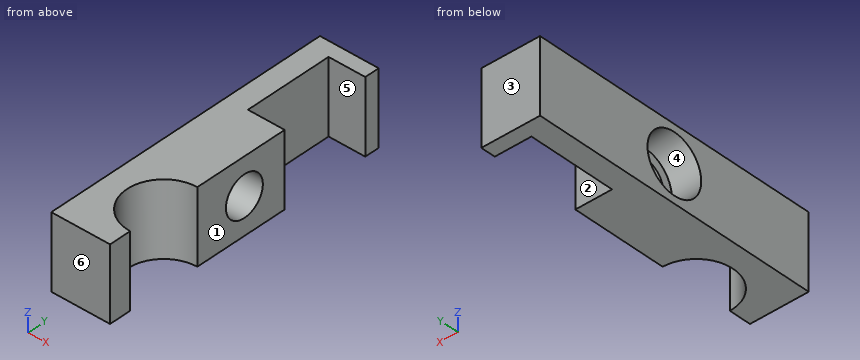
Autodesk Inventor part; units mm, degrees
ref_plane "YZ Plane" through (0, 0, 0) normal (1, 0, 0) x (0, 1, 0)
ref_plane "XZ Plane" through (0, 0, 0) normal (0, 1, 0) x (-1, 0, 0)
ref_plane "XY Plane" through (0, 0, 0) normal (0, 0, 1) x (1, 0, 0)
sketch "Sketch1" plane through (0, 0, 0) normal (0, 0, 1) x (1, 0, 0)
  line L0 (0, 0) -> (4, 0)
  line L1 (4, 0) -> (4, -20)
  line L2 (4, -20) -> (0, -20)
  line L3 (0, -20) -> (0, 0)
  circle A0 centre (4, -4) radius 2.5
  circle A1 centre (4, -16) radius 2.5
  line L4 (1.5, -4) -> (1.5, -7)
  line L5 (1.5, -7) -> (1.5, -1)
  line L6 (4, -7) -> (1.5, -7)
  line L7 (1.5, -1) -> (4, -1)
  point P0 (4, -18.5)
  point P1 (4, -13.5)
  dimension "d2" = 5
  dimension "d0" = 20
  dimension "d1" = 4
  dimension "d3" = 5
  dimension "d4" = 4
  dimension "d5" = 4
  dimension "d6" = 3
  dimension "d7" = 3
extrude "Extrusion1" add sketch "Sketch1" along normal blind 5 contours L0 L1 L7 L5 L4 L6 A1 L2 L3
sketch "Sketch3" plane through (0, -20, 0) normal (-1, 0, 0) x (0, 0, 1)
  circle A0 centre (2.5, 10) radius 1.375
  line L0 (0, 0) -> (5, 0)
  line L1 (0, 20) -> (0, 0)
  dimension "d10" = 10
  dimension "d11" = 2.5
  dimension "d12" = 20
  dimension "d13" = 2.75
extrude "Extrusion2" cut sketch "Sketch3" against normal blind 20
sketch "Sketch4" plane through (0, -20, 0) normal (-1, 0, 0) x (0, 0, 1)
  circle A0 centre (2.5, 10) radius 1.375
  circle A1 centre (2.5, 10) radius 2
  point P0 (0, 20)
  dimension "d16" = 4
extrude "Extrusion3" cut sketch "Sketch4" against normal blind 2 contours A0 | A1
equation "\"d1\" = d4"
properties part number "POMSliderAxis"
Input: part model. Units: mm. Frame: model coordinates. Face numbers are marked on the shaded views. A direction names the side the tool comes from. Give positions to 0.01 mm unless a question says otherwise; leave off trailing zeros. Write each loop counter-clockwise with the first axis right and the second up, starting at its lowest first coordinate (ties: lowest second). Pieces come first, ordered by that corner, then holes. Notation, with made-up numbers: M -12,56.5 L 44,56.5 A33 ccw 44,84.5 Z; hole C 78.5,61 d1. An arc over 180 degrees is marked long. Use one line per item in the form item = value.
1. Cut plane B-B on y = -10. Return loops of the section in (x, z) (3 decimals), and give its area (3 significant figures).
Outcome:
outline = M 0,0 L 4,0 L 4,1.125 L 2,1.125 L 2,0.5 L 0,0.5 Z; M 0,4.5 L 2,4.5 L 2,3.875 L 4,3.875 L 4,5 L 0,5 Z
area = 6.50 mm²
2. Cut plane A-A on z = 2.5. Return loops of the section in (x, y) (3 decimals), and give its area (3 significant figures).
Outcome:
outline = M 0,-20 L 4,-20 L 4,-18.5 A2.5 cw 4,-13.5 L 4,-11.375 L 2,-11.375 L 2,-12 L 0,-12 Z; M 0,-8 L 2,-8 L 2,-8.625 L 4,-8.625 L 4,-7 L 1.5,-7 L 1.5,-1 L 4,-1 L 4,0 L 0,0 Z
area = 41.7 mm²
3. Mould query, pull axis Y, two halves, no side actions, for the marked faces 1, 2 and 3. Classes: released by +Y, released by -Y, zero draft, split by the parting line, or undercut.
Outcome:
face_1 = zero draft
face_2 = undercut
face_3 = released by +Y
4. Cut plane C-C on x = 3.5. Return loops of the section in (y, z) (3 decimals).
Outcome:
outline = M -20,0 L -18.449,0 L -18.449,5 L -20,5 Z; M -13.551,0 L -7,0 L -7,5 L -13.551,5 Z; M -1,0 L 0,0 L 0,5 L -1,5 Z; hole C -10,2.5 d2.75
5. Ray query, L1, parallel to Y at x = 0.7, z = 2.5; L2, parallel to Y at x = 3.15, z = 3; L3, parallel to Y at x = 2.45, z = 4.75. Return the intervals inside material, ascending.
Outcome:
L1 = -20 to -12, -8 to 0
L2 = -20 to -18.35, -13.65 to -11.28, -8.72 to -7, -1 to 0
L3 = -20 to -17.96, -14.04 to -7, -1 to 0
6. Reachability of the marked faces 4, 5 and 6 from +Z, -Z, +X, -X, +Y, -Y: full face, straight path, thin tool, end or side. Return the list, or none.
Outcome:
face_4 = -X
face_5 = +Z, -Z, +X
face_6 = +Z, -Z, +X, -X, -Y
7. Cut plane D-D on x = 1.8. Return loops of the section in (y, z), and give its area (3 significant figures).
Outcome:
outline = M -20,0 L -17.19,0 L -17.19,5 L -20,5 Z; M -14.81,0 L -7,0 L -7,5 L -14.81,5 Z; M -1,0 L 0,0 L 0,5 L -1,5 Z; hole C -10,2.5 d4
area = 45.6 mm²
